from build123d import *

# Parameters (mm, degrees)
BOSS_EXTRUDE4_DEPTH     = 19
SKETCH1_R               = 22.5
SKETCH1_R_2             = 16.9
BOSS_EXTRUDE4_2_DEPTH   = 19
BOSS_EXTRUDE5_DEPTH     = 9
CUT_EXTRUDE1_DEPTH      = 4
FILLET1_R               = 1
FILLET2_R               = 22.5
FILLET3_R               = 40
BOSS_EXTRUDE6_DEPTH     = 30
CUT_EXTRUDE2_DEPTH      = 209.505251732
CUT_EXTRUDE2_DEPTH_BACK = 209.505251732
SKETCH6_R               = 26
CUT_EXTRUDE3_DEPTH      = 201.224099449
CUT_EXTRUDE3_DEPTH_BACK = 201.224099449
SKETCH7_R               = 4.5


with BuildPart() as part:
    # Sketch1 → Boss-Extrude4 (new, symmetric)
    with BuildSketch(Plane.XY):
        with BuildLine():
            Line((-35.026029259, -192.882712321), (-35.389042583, -194.595784299))
            ThreePointArc((-35.389042583, -194.595784299), (-35.846935246, -197.883792302), (-36, -201.2))
            Line((-36, -201.2), (-26, -201.2))
            ThreePointArc((-26, -201.2), (0, -175.2), (26, -201.2))
            Line((26, -201.2), (36, -201.2))
            ThreePointArc((36, -201.2), (35.846935246, -197.883792302), (35.389042583, -194.595784299))
            Line((35.389042583, -194.595784299), (35.026029259, -192.882712321))
            ThreePointArc((35.026029259, -192.882712321), (0, -165.2), (-35.026029259, -192.882712321))
        make_face()
    extrude(amount=BOSS_EXTRUDE4_DEPTH, both=True)



with BuildPart() as body_2:
    # Sketch1 → Boss-Extrude4 2 (new, symmetric)
    with BuildSketch(Plane.XY):
        Circle(SKETCH1_R)
        Circle(SKETCH1_R_2, mode=Mode.SUBTRACT)
    extrude(amount=BOSS_EXTRUDE4_2_DEPTH, both=True)


with BuildPart() as part_1:
    add(part.part)

    add(body_2.part)  # Boss-Extrude5 merges body 2
    # Sketch1<7> → Boss-Extrude5 (add, symmetric)
    with BuildSketch(Plane.XY):
        with BuildLine():
            Line((-10, -20.155644371), (-17.849697213, -169.936789841))
            ThreePointArc((-17.849697213, -169.936789841), (0, -165.2), (17.849697213, -169.936789841))
            Line((17.849697213, -169.936789841), (10, -20.155644371))
            ThreePointArc((10, -20.155644371), (0, -22.5), (-10, -20.155644371))
        make_face()
    extrude(amount=BOSS_EXTRUDE5_DEPTH, both=True)

    # Sketch2 → Cut-Extrude1 (cut)
    with BuildSketch(Plane.XY.offset(9)):
        with BuildLine():
            Line((8, -51.932208026), (8, -141.932208026))
            ThreePointArc((8, -141.932208026), (0, -149.932208026), (-8, -141.932208026))
            Line((-8, -141.932208026), (-8, -51.932208026))
            ThreePointArc((-8, -51.932208026), (0, -43.932208026), (8, -51.932208026))
        make_face()
    cut_extrude1 = extrude(amount=-CUT_EXTRUDE1_DEPTH, mode=Mode.SUBTRACT)

    # Mirror1: Cut-Extrude1 across plane
    add(cut_extrude1.mirror(Plane.XY), mode=Mode.SUBTRACT)

    # Fillet1
    fillet1_edges = [part_1.edges().sort_by_distance(p)[0] for p in [
        (0, -43.932208026, 5),
        (8, -96.932208026, 5),
        (0, -149.932208026, 5),
        (-8, -96.932208026, 5),
        (0, -43.932208026, 9),
        (-8, -96.932208026, 9),
        (0, -149.932208026, 9),
        (8, -96.932208026, 9),
        (0, -43.932208026, -9),
        (-8, -96.932208026, -9),
        (0, -149.932208026, -9),
        (8, -96.932208026, -9),
        (0, -43.932208026, -5),
        (-8, -96.932208026, -5),
        (0, -149.932208026, -5),
        (8, -96.932208026, -5),
    ]]
    fillet(fillet1_edges, radius=FILLET1_R)

    # Fillet2
    fillet2_edges = [part_1.edges().sort_by_distance(p)[0] for p in [
        (10, -20.155644371, 0),
        (-10, -20.155644371, 0),
    ]]
    fillet(fillet2_edges, radius=FILLET2_R)

    # Fillet3
    fillet3_edges = [part_1.edges().sort_by_distance(p)[0] for p in [
        (-17.849697213, -169.936789841, 0),
        (17.849697213, -169.936789841, 0),
    ]]
    fillet(fillet3_edges, radius=FILLET3_R)

    # Sketch3 → Boss-Extrude6 (add)
    with BuildSketch(Plane(origin=(0, -171.2, 0), x_dir=(1, 0, 0), z_dir=(0, 1, 0))):
        with BuildLine():
            Line((-38, 9), (38, 9))
            ThreePointArc((38, 9), (47, 0), (38, -9))
            Line((38, -9), (-38, -9))
            ThreePointArc((-38, -9), (-47, 0), (-38, 9))
        make_face()
    extrude(amount=-BOSS_EXTRUDE6_DEPTH)

    # Sketch6 → Cut-Extrude2 (cut, two sides: drawn at the far end of the back side and taken through both)
    with BuildSketch(Plane.XY.offset(9).offset(-CUT_EXTRUDE2_DEPTH_BACK)):
        with Locations((0, -201.2)):
            Circle(SKETCH6_R)
    extrude(amount=CUT_EXTRUDE2_DEPTH + CUT_EXTRUDE2_DEPTH_BACK, mode=Mode.SUBTRACT)

    # Sketch7 → Cut-Extrude3 (cut, two sides: drawn at the far end of the back side and taken through both)
    with BuildSketch(Plane(origin=(0, -171.2, 0), x_dir=(1, 0, 0), z_dir=(0, 1, 0)).offset(-CUT_EXTRUDE3_DEPTH_BACK)):
        with Locations(Location((-38, 0, 0), (0, 0, 270))):
            Circle(SKETCH7_R)
        with Locations(Location((38, 0, 0), (0, 0, 270))):
            Circle(SKETCH7_R)
    extrude(amount=CUT_EXTRUDE3_DEPTH + CUT_EXTRUDE3_DEPTH_BACK, mode=Mode.SUBTRACT)


solid = part_1.part
For this review, take the finished solid that the model builds, in its own axes (mm). A direction names the side the tool comes from. Round coordinates to 2 decimals unless told otherwise and drop trailing zeros. Write each loop counter-clockwise with the first axis right and the second up, starting at its lowest first coordinate (ties: lowest second). Pieces come first, ordered by that corner, then holes. Notation, with made-up numbers: (83, 54.25) - (106, 54.25) arc R26 cw to (106, 80.25) - close; hole circle Ø5 at (23.25, 39). An arc over 180 degrees is marked (long way). Write item = value, one per line. Start each with the question number.
1. Wall thickness on L1, parallel to Y at x = 0, z = 10; L2, parallel to Y at x = 0, z = 8; L3, parallel to Z at x = -38, y = -191.75: over which ranges is each line inside the solid? List them lowest first.
2. Consider section C-C on y = 0. State the section outline as (x, z) points, plus the area to 3 significant figures.
3. For faces 1 (the face through (-0.176, -43.934, 7.014)), 2 (the face through (-18.574, -162.262, 0.126)), 3 (the face through (-35.843, -197.837, -13.93)), 4 (the face through (13.826, -93.152, 0.126)), list the 3-axis set-ups (+Z, -Z, +X, -X, +Y, -Y) from which the entire face can be reached by the end or side of a thin tool; tool diameter is ignored.
4. For pin 1 Ø2 at (y, z) = (-31.5, -6) entering from +X; pin 2 Ø12 at (y, z) = (-47, -0.5) entering from -X; pin 3 Ø12 at (y, z) = (-16, -4) entering from +X, all flat-tipped, find the tip position at first contact; note any pin that passes through.
5. Consider section D-D on y = -183. State the section outline as (x, z) points.
6. Consider section A-A on z = 0. State the section outline as (x, y) points.
7. Draft analysis for pull direction X (two halves, no side actions). For faces 5 (the face through (33.61, -186.41, -0.98)), 6 (the face through (-1, -175, -19)), 7 (the face through (-35.843, -197.837, 14.07)), 8 (the face through (35.85, -197.93, -13.93)), state which applies: released by +X, released by -X, zero draft, split by the parting line, or undercut.
Evaluation:
q1.L1 = -175.2 to -165.2, -22.5 to -16.9, 16.9 to 22.5
q1.L2 = -175.2 to -149.93, -43.93 to -16.9, 16.9 to 22.5
q1.L3 = -9 to -4.5, 4.5 to 9
q2.outline = (-22.5, -19) - (-16.9, -19) - (-16.9, 19) - (-22.5, 19) - close; (16.9, -19) - (22.5, -19) - (22.5, 19) - (16.9, 19) - close
q2.area = 426 mm2
q3.face_1 = +Z
q3.face_2 = +Z, -Z, -X
q3.face_3 = -Z, -X, +Y
q3.face_4 = +Z, -Z, +X
q4.pin_1 = 10.65
q4.pin_2 = -11.72
q4.pin_3 = 20.16
q5.outline = (-38, -9) - (-31.06, -9) - (-31.06, -19) - (-18.57, -19) - (-18.57, 19) - (-31.06, 19) - (-31.06, 9) - (-38, 9) arc R9 ccw to start; (18.57, -19) - (31.06, -19) - (31.06, -9) - (38, -9) arc R9 ccw to (38, 9) - (31.06, 9) - (31.06, 19) - (18.57, 19) - close; hole circle Ø9 at (-38, 0); hole circle Ø9 at (38, 0)
q6.outline = (-47, -201.2) - (-42.5, -201.2) - (-42.5, -171.2) - (-47, -171.2) - close; (-33.5, -201.2) - (-26, -201.2) arc R26 cw to (26, -201.2) - (33.5, -201.2) - (33.5, -171.2) - (22.48, -171.2) arc R40 cw to (16.96, -152.91) - (10.6, -31.69) arc R22.5 cw to (16.54, -15.26) arc R22.5 ccw (long way) to (-16.54, -15.26) arc R22.5 cw to (-10.6, -31.69) - (-16.96, -152.91) arc R40 cw to (-22.48, -171.2) - (-33.5, -171.2) - close; (42.5, -201.2) - (47, -201.2) - (47, -171.2) - (42.5, -171.2) - close; hole circle Ø33.8 at (0, 0)
q7.face_5 = undercut
q7.face_6 = zero draft
q7.face_7 = released by -X
q7.face_8 = released by +X
